```python
from build123d import *

# Parameters (mm, degrees)
F0_W     = 127
F0_H     = 76.2
F1_DEPTH = 12.7
F2_W     = 25.4
F2_H     = 33.5525823757
F3_DEPTH = 38.1
F4_W     = 17.7103555709
F4_H     = 19.1524197951
F5_DEPTH = 25.401
F6_R     = 28.3213454148
F7_DEPTH = 12.701


with BuildPart() as f1:
    # F0 (on Top) → F1 (new body)
    with BuildSketch(Plane.XY):
        Rectangle(F0_W, F0_H)
        with BuildLine():
            Line((-63.5, -38.1), (-63.5, 38.1))
            ThreePointArc((-63.5, 38.1), (-115.2096482651, 0), (-63.5, -38.1))
        make_face()
    extrude(amount=F1_DEPTH)

    # F2 (on Front) → F3 (join, symmetric)
    with BuildSketch(Plane.XZ):
        with Locations((50.8, 29.4762911879)):
            Rectangle(F2_W, F2_H)
    extrude(amount=F3_DEPTH, both=True)

    # F4 (on face) → F5 (cut, through all)
    with BuildSketch(Plane(origin=(38.1, 0, 0), x_dir=(0, -1, 0), z_dir=(-1, 0, 0))):
        with Locations((29.2448222145, 36.6763724782)):
            Rectangle(F4_W, F4_H)
    extrude(amount=-F5_DEPTH, mode=Mode.SUBTRACT)

    # F6 (on face) → F7 (cut, through all)
    with BuildSketch(Plane.XY.offset(12.7)):
        with Locations((-8.5171926767, 0)):
            Circle(F6_R)
    extrude(amount=-F7_DEPTH, mode=Mode.SUBTRACT)


solid = f1.part
```
Input: part model. Units: mm. Frame: model coordinates. A direction names the side the tool comes from. Round coordinates to 2 decimals unless told otherwise and drop trailing zeros. Loops run counter-clockwise (first coordinate to the right, second up) from the corner with the lowest first, then second, coordinate; pieces in that order, holes last. Notation, with made-up numbers: (79.5, 33) -> (120.5, 33) arc R9 cw to (120.5, 44) -> close; hole circle Ø11 at (69, 4). An arc over 180 degrees is marked (long way). Use one line per item in the form item = value. Start each with the question number.
Item 1: Set-up query: faces 1 (the face through (-47, 1, 0)), 2 (the face through (-40, 1, 12.7)), 3 (the face through (51, -20.39, 37)). Return all of +Z, -Z, +X, -X, +Y, -Y with unobstructed straight access to the full face (end or side cutting, diameter ignored); none if empty.
Item 2: Section query B-B on z = 6. Return the cut outline in (x, y), then the cut area to 3 significant figures.
Item 3: Contact query for flat-ended pins moving along their axis: pin 1 Ø3 at (y, z) = (-3.5, 18.5) entering from -X; pin 2 Ø9.5 at (x, z) = (48.5, 33.5) entering from -Y; pin 3 Ø13.5 at (x, z) = (5.5, 17) entering from -Y; pin 4 Ø5 at (x, y) = (-40, -12) entering from -Z. Output: stop coordinate, or through.
Item 4: Section query C-C on x = -5. Return the cut outline in (y, z).
Item 5: Section query D-D on y = 12. Return the cut outline in (x, z), then the cut area to 3 significant figures.
Item 6: Mould query, pull axis Y, two halves, no side actions, for faces 4 (the face through (18.5, 8.5, 6.4)), 5 (the face through (-115.196, 1.045, 6.261)), 6 (the face through (27, 38.1, 8)), 7 (the face through (13, -38.1, 8)). Classes: pulls with the +Y half, pulls with the -Y half, needs draft (parallel to the pull), parting line crosses it, or undercut.
Item 7: Section query A-A on y = 0. Return the cut outline in (x, z), then the cut area to 3 significant figures.
Item 8: Material intervals for L1, parallel to X at y = -10, z = 41; L2, parallel to Z at x = -73.5, y = -27; L3, parallel to Y at x = 27, z = 5, sorted ascending. Write a range as from..to.
Ans:
q1.face_1 = -Z, +X, -X, +Y, -Y
q1.face_2 = +Z, -X, +Y, -Y
q1.face_3 = +Z, +X, -X, -Y
q2.outline = (-63.5, -38.1) -> (63.5, -38.1) -> (63.5, 38.1) -> (-63.5, 38.1) arc R39.89 ccw (long way) to start; hole circle Ø56.64 at (-8.52, 0)
q2.area = 10,600 mm^2
q3.pin_1 = 38.1
q3.pin_2 = -20.39
q3.pin_3 = -38.1
q3.pin_4 = 0
q4.outline = (-38.1, 0) -> (-28.1, 0) -> (-28.1, 12.7) -> (-38.1, 12.7) -> close; (28.1, 0) -> (38.1, 0) -> (38.1, 12.7) -> (28.1, 12.7) -> close
q5.outline = (-113.36, 0) -> (-34.17, 0) -> (-34.17, 12.7) -> (-113.36, 12.7) -> close; (17.14, 0) -> (63.5, 0) -> (63.5, 46.25) -> (38.1, 46.25) -> (38.1, 12.7) -> (17.14, 12.7) -> close
q5.area = 2,450 mm^2
q6.face_4 = undercut
q6.face_5 = parting line crosses it
q6.face_6 = pulls with the +Y half
q6.face_7 = pulls with the -Y half
q7.outline = (-115.21, 0) -> (-36.84, 0) -> (-36.84, 12.7) -> (-115.21, 12.7) -> close; (19.8, 0) -> (63.5, 0) -> (63.5, 46.25) -> (38.1, 46.25) -> (38.1, 12.7) -> (19.8, 12.7) -> close
q7.area = 2,400 mm^2
q8.L1 = 38.1..63.5
q8.L2 = 0..12.7
q8.L3 = -38.1..38.1
